from build123d import *

# Parameters (mm, degrees)
BOSS_EXTRUDE1_DEPTH = 20
SKETCH3_W           = 15
SKETCH3_H           = 5
CUT_EXTRUDE2_DEPTH  = 8
SKETCH4_R           = 2
CUT_EXTRUDE3_DEPTH  = 110
SKETCH2_R           = 2
CUT_EXTRUDE4_DEPTH  = 110
SKETCH5_W           = 43
SKETCH5_H           = 27
BOSS_EXTRUDE2_DEPTH = 5
SKETCH6_W           = 40
SKETCH6_H           = 20.5
CUT_EXTRUDE5_DEPTH  = 5
FILLET1_R           = 0.5
BOSS_EXTRUDE3_DEPTH = 62.5
SKETCH8_R           = 3
CUT_EXTRUDE6_DEPTH  = 62.5


with BuildPart() as part:
    # Sketch1 → Boss-Extrude1 (new body)
    with BuildSketch(Plane.XY):
        Polygon((0, 0), (12.551397955, 0), (12.551397955, 19.52439682), (70, 19.52439682), (70, 24.52439682), (12.551397955, 24.52439682), (12.551397955, 49.048793639), (0, 49.048793639), (0, 52.048793639), (-10, 52.048793639), (-10, 41.048793639), (0, 41.048793639), (0, 44.048793639), (7.551397955, 44.048793639), (7.551397955, 24.52439682), (7.551397955, 5), (0, 5), (0, 8), (-10, 8), (-10, -3), (0, -3), align=None)
    extrude(amount=BOSS_EXTRUDE1_DEPTH)

    # Sketch3 → Cut-Extrude2 (cut)
    with BuildSketch(Plane.ZY.offset(10)):
        with Locations((10, 2.5)):
            Rectangle(SKETCH3_W, SKETCH3_H)
    cut_extrude2 = extrude(amount=-CUT_EXTRUDE2_DEPTH, mode=Mode.SUBTRACT)

    # Mirror1: Cut-Extrude2 across plane
    add(cut_extrude2.mirror(Plane(origin=(12.551397955, 24.52439682, 20), x_dir=(0, 0, 1), z_dir=(0, -1, 0))), mode=Mode.SUBTRACT)

    # Sketch4 → Cut-Extrude3 (cut)
    with BuildSketch(Plane(origin=(0, 52.048793639, 0), x_dir=(1, 0, 0), z_dir=(0, 1, 0))):
        with Locations((-5, -5)):
            Circle(SKETCH4_R)
        with Locations((-5, -15)):
            Circle(SKETCH4_R)
    extrude(amount=-CUT_EXTRUDE3_DEPTH, mode=Mode.SUBTRACT)

    # Sketch2 → Cut-Extrude4 (cut)
    with BuildSketch(Plane.XZ.offset(-19.52439682)):
        with Locations((66, 15)):
            Circle(SKETCH2_R)
        with Locations((18, 15)):
            Circle(SKETCH2_R)
        with Locations((18, 5)):
            Circle(SKETCH2_R)
        with Locations((66, 5)):
            Circle(SKETCH2_R)
    extrude(amount=-CUT_EXTRUDE4_DEPTH, mode=Mode.SUBTRACT)

    # Sketch5 → Boss-Extrude2 (add)
    with BuildSketch(Plane.XZ.offset(-19.52439682)):
        with Locations((42, 10)):
            Rectangle(SKETCH5_W, SKETCH5_H)
    extrude(amount=-BOSS_EXTRUDE2_DEPTH)

    # Sketch6 → Cut-Extrude5 (cut)
    with BuildSketch(Plane.XZ.offset(-19.52439682)):
        with Locations((42, 10)):
            Rectangle(SKETCH6_W, SKETCH6_H)
    extrude(amount=-CUT_EXTRUDE5_DEPTH, mode=Mode.SUBTRACT)

    # Fillet1
    fillet1_edges = [part.edges().sort_by_distance(p)[0] for p in [
        (63.5, 22.02439682, 23.5),
        (63.5, 22.02439682, -3.5),
        (20.5, 22.02439682, -3.5),
        (20.5, 22.02439682, 23.5),
        (62, 22.02439682, 20.25),
        (62, 22.02439682, -0.25),
        (22, 22.02439682, -0.25),
        (22, 22.02439682, 20.25),
    ]]
    fillet(fillet1_edges, radius=FILLET1_R)

    # Sketch7 → Boss-Extrude3 (add)
    with BuildSketch(Plane(origin=(70, 0, 0), x_dir=(0, 0, -1), z_dir=(1, 0, 0))):
        Polygon((0, 19.52439682), (3.5, 19.52439682), (3.5, 51.958822175), (-20, 52.048793639), (-20, 49.048793639), (0, 49.048793639), align=None)
    extrude(amount=-BOSS_EXTRUDE3_DEPTH)

    # Sketch8 → Cut-Extrude6 (cut)
    with BuildSketch(Plane(origin=(0, 51.971460384, -0.198976528), x_dir=(1, 0, 0), z_dir=(0, 0.999992671, -0.003828545))):
        with Locations((53.5, -10.198952335)):
            Circle(SKETCH8_R)
    extrude(amount=-CUT_EXTRUDE6_DEPTH, mode=Mode.SUBTRACT)


solid = part.part
Verification items for the finished model (mm, model axes). A direction names the side the tool comes from. Give positions to 0.01 mm unless a question says otherwise; leave off trailing zeros. Write each loop counter-clockwise with the first axis right and the second up, starting at its lowest first coordinate (ties: lowest second). Pieces come first, ordered by that corner, then holes.
(1) Gauge pin test, flat ends, axial feed: pin 1 (2.5 mm diameter, centred on y = 22.5, z = 21.5, fed in from +X); pin 2 (2.5 mm diameter, centred on x = -7.5, y = 47.5, fed in from +Z); pin 3 (1.5 mm diameter, centred on x = 22.5, z = 7, fed in from +Y). Record the tip position at first contact, or that the pin passes through.
(2) Cross-section at B-B (y = 48). Enter the section's corners in (x, z).
(3) Access from +Z, -Z, +X, -X, +Y, -Y to the whole of each face (thin tool, end or side, straight path). Record for faces 4 (the face through (66, 22, 17)), 5 (the face through (0, 43, 10)), 6 (the face through (-6, 2, 2.5)), 7 (the face through (37, 24.524, 21)).
(4) Mould release check, pull along X, two halves, no side actions. Record for faces 1 (the face through (-5, -1, 13)), 2 (the face through (-10, 6, 10)), 3 (the face through (41, 19.524, -1)): +X half, -X half, draft (parallel to the pull), parting line (faces both ways), or undercut.
(5) Material ranges on line 1 (Y direction, x = -5.5, z = 10); line 2 (Z direction, x = -5, y = 42.35); line 3 (X direction, y = 49.5, z = 10.25), recorded low to high.
(6) Cross-section at D-D (x = 38.5). Enter the section's corners in (y, z).
(7) Cross-section at A-A (x = 4). Enter the section's corners in (y, z).
(8) Cross-section at C-C (x = 18). Enter the section's corners in (y, z).
Worked out:
1. pin 1: stops at x = 63.5
1. pin 2: stops at z = 20
1. pin 3: stops at y = 52
2. outline: (-10, 0) - (7.5, 0) - (7.5, -3.5) - (70, -3.5) - (70, 0) - (12.55, 0) - (12.55, 20) - (-10, 20) - (-10, 17.5) - (-2, 17.5) - (-2, 2.5) - (-10, 2.5) - close
3. face 4: -Y
3. face 5: +Z, -Z
3. face 6: -X
3. face 7: +Z, +X
4. face 1: undercut
4. face 2: -X half
4. face 3: draft
5. line 1: y = -3 to 0, 5 to 8, 41.05 to 44.05, 49.05 to 52.05
5. line 2: z = 0 to 3, 7 to 13, 17 to 20
5. line 3: x = -10 to 0, 7.5 to 50.51, 56.49 to 70
6. outline: (19.52, -3.5) - (51.96, -3.5) - (52.05, 20) - (49.05, 20) - (49.05, 0) - (19.52, 0) - close; (19.52, 20.25) - (24.52, 20.25) - (24.52, 23.5) - (19.52, 23.5) - close
7. outline: (0, 0) - (5, 0) - (5, 20) - (0, 20) - close; (44.05, 0) - (49.05, 0) - (49.05, 20) - (44.05, 20) - close
8. outline: (19.52, -3.5) - (51.96, -3.5) - (52.05, 20) - (49.05, 20) - (49.05, 0) - (24.52, 0) - (24.52, 3) - (19.52, 3) - close; (19.52, 7) - (24.52, 7) - (24.52, 13) - (19.52, 13) - close; (19.52, 17) - (24.52, 17) - (24.52, 20) - (19.52, 20) - close
